Job drawing, mm, ordinate dimensions from the low corner. One solid piece. A direction names the side the tool comes from. Give positions to 0.01 mm unless a question says otherwise; leave off trailing zeros. Order: outer loops, then holes, each group sorted by start corner. A loop starts at its lowest first (then second) coordinate and runs counter-clockwise, first axis right, second up.
Item 1: Band-saw the part on B-B on z = 4.5. Give the cut face in (x, y).
Item 2: Band-saw the part on A-A on y = 7. Give the cut face in (x, z), plus the area to 3 significant figures.
Item 3: Which spindle directions (+Z, -Z, +X, -X, +Y, -Y) get a long thin tool onto all of the face, cutting with end or side? Do the marked faces 1, 2 and 3. Say none if no direction does.
Item 4: Flat gauge pins, fed straight in: P1, Ø4.5, axis at y = 25.5, z = 4, coming from the -X side; P2, Ø1, axis at x = 5, y = 7.5, coming from the -Z side; P3, Ø3, axis at y = 24.5, z = 2, coming from the +X side. Where does each tip first touch, or does it go through?
Item 5: Band-saw the part on D-D on z = 7. Give the cut face in (x, y).
Item 6: Wall check: L1, parallel to Y at x = 2.65, z = 4.5; L2, parallel to Y at x = 3.35, z = 4.5; L3, parallel to X at y = 11, z = 4.25. Give the ranges that are in metal, low to high.
Item 7: Band-saw the part on C-C on x = 31. Give the cut face in (y, z), plus the area to 3 significant figures.
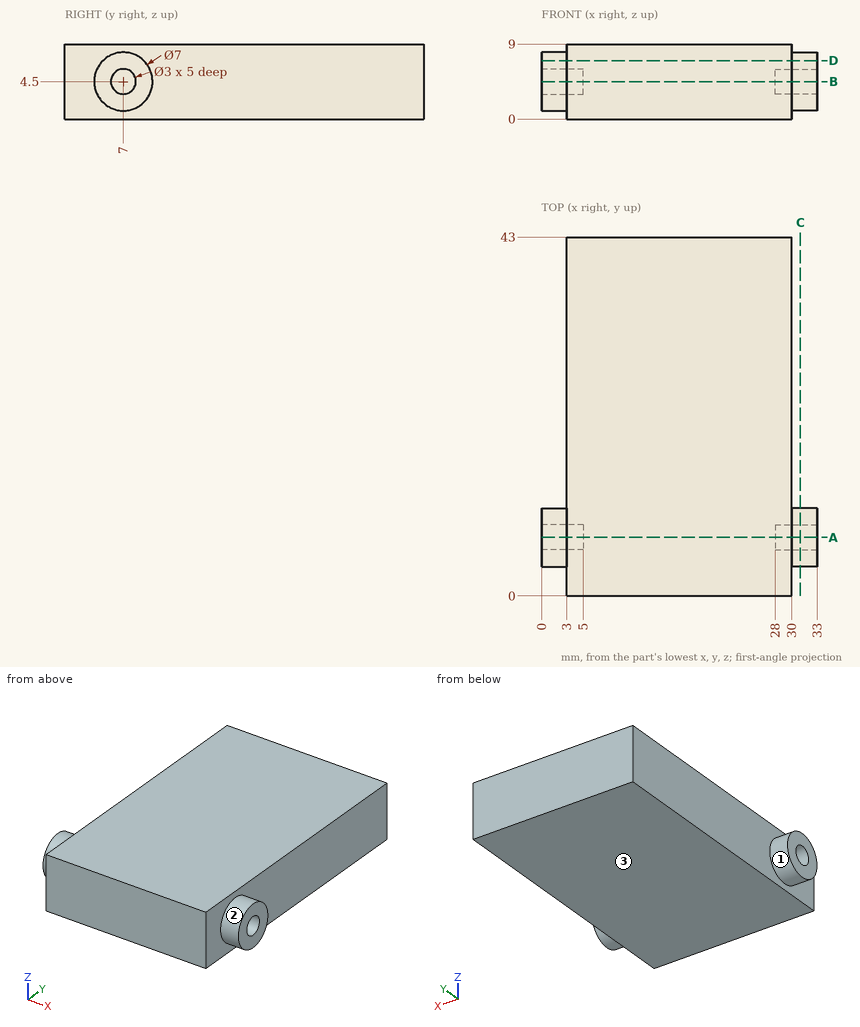
The answers:
1. outline: (0, 3.5) - (3, 3.5) - (3, 0) - (30, 0) - (30, 3.5) - (33, 3.5) - (33, 5.5) - (28, 5.5) - (28, 8.5) - (33, 8.5) - (33, 10.5) - (30, 10.5) - (30, 43) - (3, 43) - (3, 10.5) - (0, 10.5) - (0, 8.5) - (5, 8.5) - (5, 5.5) - (0, 5.5) - close
2. outline: (0, 1) - (3, 1) - (3, 0) - (30, 0) - (30, 1) - (33, 1) - (33, 3) - (28, 3) - (28, 6) - (33, 6) - (33, 8) - (30, 8) - (30, 9) - (3, 9) - (3, 8) - (0, 8) - (0, 6) - (5, 6) - (5, 3) - (0, 3) - close
2. area: 255 mm2
3. face 1: -X
3. face 2: +X
3. face 3: -Z, +X, -X, +Y, -Y
4. P1: stops at x = 3
4. P2: stops at z = 0
4. P3: stops at x = 30
5. outline: (0, 4.55) - (3, 4.55) - (3, 0) - (30, 0) - (30, 4.55) - (33, 4.55) - (33, 9.45) - (30, 9.45) - (30, 43) - (3, 43) - (3, 9.45) - (0, 9.45) - close
6. L1: y = 3.5 to 5.5, 8.5 to 10.5
6. L2: y = 0 to 5.5, 8.5 to 43
6. L3: x = 3 to 30
7. outline: circle Ø7 at (7, 4.5); hole circle Ø3 at (7, 4.5)
7. area: 31.4 mm2
